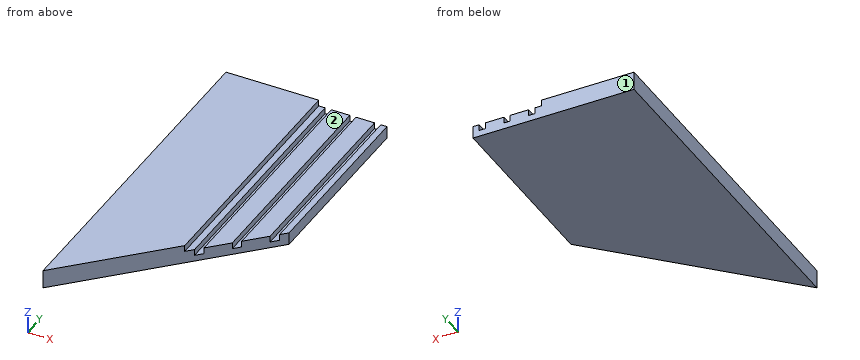
from build123d import *

# Parameters (mm, degrees)
F0_W        = 30
F0_H        = 10
F0_W_2      = 10.3326633751
F1_DEPTH    = 300
F2_T1_DEPTH = 1563.0097927795


# Not quite as in the source:
# - a fillet or chamfer that OpenCascade refuses, or shapes differently, is made with other operations: its cross-section is extruded or revolved along the edge and cut away or added


with BuildPart() as f1:
    # F0 (on Front) → F1 (new body, symmetric)
    with BuildSketch(Plane.XZ):
        Polygon((-41.8675842226, -17.4409984683), (-41.8675842226, -7.4409984683), (-191.8675842226, -7.4409984683), (-191.8675842226, -37.4409984683), (-41.8675842226, -37.4409984683), (-41.8675842226, -27.4409984683), align=None)
        with Locations((33.4650791525, -22.4409984683)):
            Rectangle(F0_W, F0_H)
        with Locations((-36.7012525351, -22.4409984683)):
            Rectangle(F0_W_2, F0_H)
        with Locations((-6.5349208475, -22.4409984683)):
            Rectangle(F0_W, F0_H)
        Polygon((-31.5349208475, -27.4409984683), (-41.8675842226, -27.4409984683), (-41.8675842226, -37.4409984683), (58.5501386541, -37.4409984683), (58.5501386541, -27.4409984683), (48.4650791525, -27.4409984683), (18.4650791525, -27.4409984683), (8.4650791525, -27.4409984683), (-21.5349208475, -27.4409984683), align=None)
        Polygon((58.5501386541, -27.4409984683), (58.5501386541, -37.4409984683), (68.5501386541, -37.4409984683), (68.5501386541, -17.4409984683), (58.5501386541, -17.4409984683), align=None)
    extrude(amount=F1_DEPTH, both=True)

    # F2: chamfer of 300 on 1 edges, made by hand

    # F2_s2 → F2_t1 (cut)
    with BuildSketch(Plane.XY.offset(-808.945894858)):
        Polygon((68.5501386541, 0), (-231.4498613459, -300), (68.5501386541, -300), align=None)
    extrude(amount=F2_T1_DEPTH, mode=Mode.SUBTRACT)


solid = f1.part
CAD build for the part. Positions are in the model's coordinates, mm. Face numbers are marked on the shaded views. A direction names the side the tool comes from. Give positions to 0.01 mm unless a question says otherwise; leave off trailing zeros. Write each loop counter-clockwise with the first axis right and the second up, starting at its lowest first coordinate (ties: lowest second). Pieces come first, ordered by that corner, then holes. Notation, with made-up numbers: M 82.5,-33 L 135.5,-33 A21 ccw 135.5,-27 Z; hole C -3.75,-21 d1. An arc over 180 degrees is marked long. Put each result on its own line as item: value. Start each with the question number.
(1) Band-saw the part on A-A, the plane y = 185.5. Write the cut outline in (x, z), and give its area (3 significant figures).
(2) Flat gauge pin, fed straight in: pin 1 Ø11 at (x, y) = (-26.5, 169) entering from +Z. Where does the tip first touch, or does it go through?
(3) Band-saw the part on C-C, the plane x = -125. Write the cut outline in (y, z).
(4) Band-saw the part on B-B, the plane z = -32.5. Write the cut outline in (x, y).
(5) Which spindle directions (+Z, -Z, +X, -X, +Y, -Y) get a long thin tool onto all of the face, cutting with end or side? Do the marked faces 1 and 2. Say none if no direction does.
(6) Probe L1, parallel to X at y = 212, z = -25.5; L2, parallel to Z at x = 44, y = 222; L3, parallel to X at y = -78, z = -14. List the from-to ranges inside material, lowest first.
Response values:
1. outline: M -191.87,-37.44 L 68.55,-37.44 L 68.55,-17.44 L 58.55,-17.44 L 58.55,-27.44 L 48.47,-27.44 L 48.47,-17.44 L 18.47,-17.44 L 18.47,-27.44 L 8.47,-27.44 L 8.47,-17.44 L -21.53,-17.44 L -21.53,-27.44 L -31.53,-27.44 L -31.53,-17.44 L -41.87,-17.44 L -41.87,-7.44 L -191.87,-7.44 Z
1. area: 6,410 mm2
2. pin 1: stops at z = -17.44
3. outline: M -193.55,-37.44 L 300,-37.44 L 300,-7.44 L -193.55,-7.44 Z
4. outline: M -191.87,-260.42 L 68.55,0 L 68.55,300 L -191.87,300 Z
5. face 1: +Z, -Z, +X, -X, +Y
5. face 2: +Z, +X, +Y, -Y
6. L1: x = -191.87 to -31.53, -21.53 to 8.47, 18.47 to 48.47, 58.55 to 68.55
6. L2: z = -37.44 to -17.44
6. L3: x = -191.87 to -41.87
